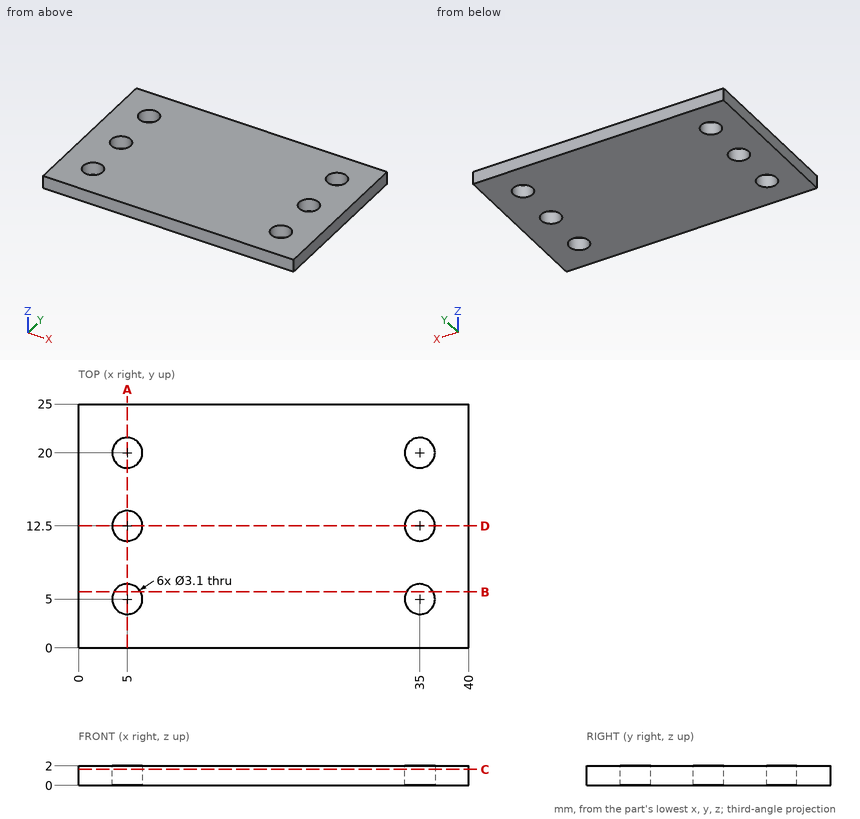
For this review, use the dimensioned drawing (mm, ordinates from the lowest corner) and the shaded views. Coordinates: 2 decimals unless noted, no trailing zeros. Write each loop counter-clockwise with the first axis right and the second up, starting at its lowest first coordinate (ties: lowest second). Pieces come first, ordered by that corner, then holes. Notation, with made-up numbers: (-29, 60.25) -> (7, 60.25) arc R23 ccw to (7, 83.25) -> close; hole circle Ø4 at (79, -3.75). An arc over 180 degrees is marked (long way). Put each result on its own line as item: value.
Q1. Take a section at A-A, the plane x = 5. State the section outline as (y, z) points.
From the geometry:
outline: (0, 0) -> (3.45, 0) -> (3.45, 2) -> (0, 2) -> close; (6.55, 0) -> (10.95, 0) -> (10.95, 2) -> (6.55, 2) -> close; (14.05, 0) -> (18.45, 0) -> (18.45, 2) -> (14.05, 2) -> close; (21.55, 0) -> (25, 0) -> (25, 2) -> (21.55, 2) -> close
Q2. Take a section at C-C, the plane z = 1.65. State the section outline as (x, y) points, then the cut area to 3 significant figures.
From the geometry:
outline: (0, 0) -> (40, 0) -> (40, 25) -> (0, 25) -> close; hole circle Ø3.1 at (5, 5); hole circle Ø3.1 at (5, 12.5); hole circle Ø3.1 at (5, 20); hole circle Ø3.1 at (35, 5); hole circle Ø3.1 at (35, 12.5); hole circle Ø3.1 at (35, 20)
area: 955 mm2
Q3. Take a section at B-B, the plane y = 5.75. State the section outline as (x, z) points, then the cut area to 3 significant figures.
From the geometry:
outline: (0, 0) -> (3.64, 0) -> (3.64, 2) -> (0, 2) -> close; (6.36, 0) -> (33.64, 0) -> (33.64, 2) -> (6.36, 2) -> close; (36.36, 0) -> (40, 0) -> (40, 2) -> (36.36, 2) -> close
area: 69.1 mm2
Q4. Wall thickness on L1, parallel to Y at x = 5, z = 0.75; L2, parallel to X at y = 5.5, z = 1.9; L3, parallel to Y at x = 34, z = 1.4: over which ranges is each line inside the solid? List them lowest first.
From the geometry:
L1: y = 0 to 3.45, 6.55 to 10.95, 14.05 to 18.45, 21.55 to 25
L2: x = 0 to 3.53, 6.47 to 33.53, 36.47 to 40
L3: y = 0 to 3.82, 6.18 to 11.32, 13.68 to 18.82, 21.18 to 25
Q5. Take a section at D-D, the plane y = 12.5. State the section outline as (x, z) points.
From the geometry:
outline: (0, 0) -> (3.45, 0) -> (3.45, 2) -> (0, 2) -> close; (6.55, 0) -> (33.45, 0) -> (33.45, 2) -> (6.55, 2) -> close; (36.55, 0) -> (40, 0) -> (40, 2) -> (36.55, 2) -> close
